Source: three-view drawing plus pictorial views. Frame: mm from the lowest corner of the part. Give positions to 0.01 mm unless a question says otherwise; leave off trailing zeros. Loops run counter-clockwise (first coordinate to the right, second up) from the corner with the lowest first, then second, coordinate; pieces in that order, holes last.
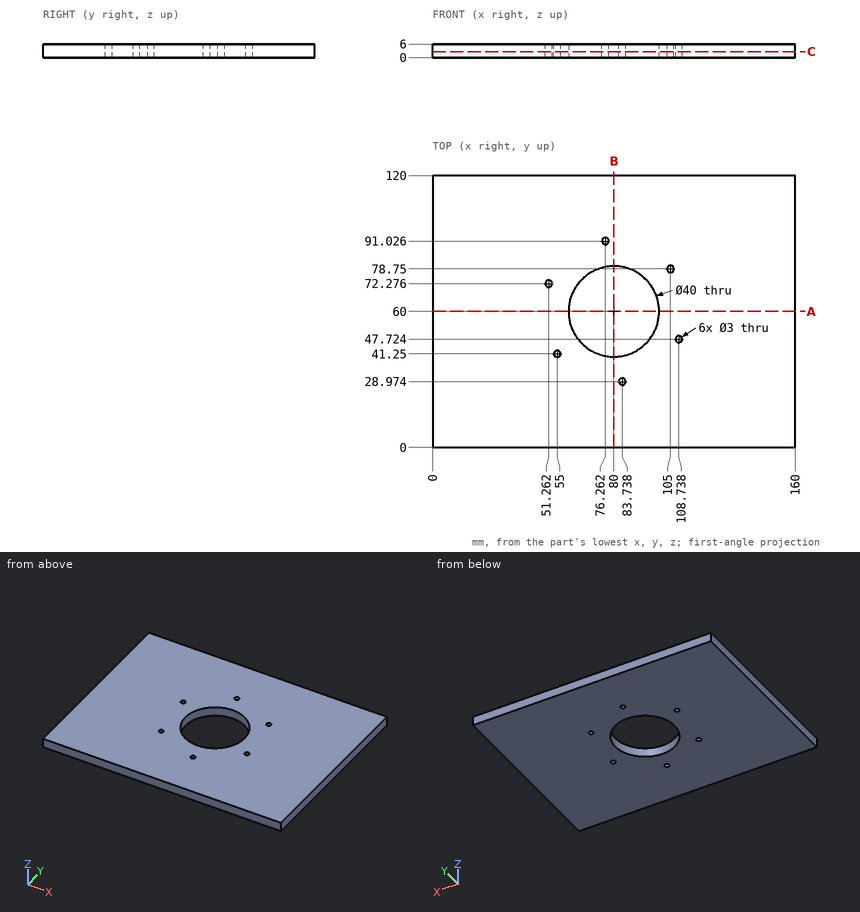
(1) Cut plane B-B (x = 80). Return the cut outline in (y, z).
Values follow:
outline: (0, 0) - (40, 0) - (40, 6) - (0, 6) - close; (80, 0) - (120, 0) - (120, 6) - (80, 6) - close
(2) Cut plane A-A (y = 60). Return the cut outline in (x, z), and give its area (3 significant figures).
Values follow:
outline: (0, 0) - (60, 0) - (60, 6) - (0, 6) - close; (100, 0) - (160, 0) - (160, 6) - (100, 6) - close
area: 720 mm2
(3) Cut plane C-C (z = 2.65). Count the separate pieces of the cut face and the enclosed holes in it, and give its area (3 significant figures).
Values follow:
separate pieces: 1
enclosed holes: 7
area: 17,900 mm2
(4) Ray query, probe 1 along Y at (x, z) = (80, 2.8); probe 2 along Y at (x, z) = (83.5, 0.7) (1 decimal); probe 3 along X at (y, z) = (78, 4.8) (1 decimal). Return the intervals inside material, ascending.
Values follow:
probe 1: y = 0 to 40, 80 to 120
probe 2: y = 0 to 27.5, 30.5 to 40.3, 79.7 to 120
probe 3: x = 0 to 71.3, 88.7 to 103.7, 106.3 to 160
